```python
from build123d import *

# Parameters (mm, degrees)
SKETCH_W        = 45
SKETCH_H        = 85
PAD_DEPTH       = 10
SKETCH001_W     = 10
SKETCH001_H     = 30
PAD001_DEPTH    = 50
SKETCH002_R     = 2.5
POCKET_DEPTH    = 10
SKETCH003_R     = 2.5
POCKET001_DEPTH = 11
POCKET002_DEPTH = 5
CHAMFER_SIZE    = 17
CHAMFER001_SIZE = 2
CHAMFER002_SIZE = 5


with BuildPart() as part:
    # Sketch → Pad (new body)
    with BuildSketch(Plane.XZ):
        Rectangle(SKETCH_W, SKETCH_H)
    extrude(amount=PAD_DEPTH)

    # Sketch001 (on Face6 of Pad) → Pad001 (join)
    with BuildSketch(Plane.XZ.offset(10)):
        with Locations((-17.5, -27.5)):
            Rectangle(SKETCH001_W, SKETCH001_H)
    extrude(amount=PAD001_DEPTH)

    # Sketch002 (on Face7 of Pad001) → Pocket (cut)
    with BuildSketch(Plane(origin=(-22.5, 0, 0), x_dir=(0, 0, -1), z_dir=(-1, 0, 0))):
        with Locations((35, 52.5)):
            Circle(SKETCH002_R)
        with Locations((35, 37.5)):
            Circle(SKETCH002_R)
    extrude(amount=-POCKET_DEPTH, mode=Mode.SUBTRACT)

    # Sketch003 (on Face5 of Pocket) → Pocket001 (cut)
    with BuildSketch(Plane.XZ.offset(10)):
        with Locations((15, 35)):
            Circle(SKETCH003_R)
        with Locations((15, 20)):
            Circle(SKETCH003_R)
    extrude(amount=-POCKET001_DEPTH, mode=Mode.SUBTRACT)

    # Sketch004 (on Face4 of Pocket001) → Pocket002 (cut)
    with BuildSketch(Plane(origin=(0, 0, 0), x_dir=(1, 0, 0), z_dir=(0, 1, 0))):
        Polygon((15, -24.75), (19.113621, -22.375), (19.113621, -17.625), (15, -15.25), (10.886379, -17.625), (10.886379, -22.375), align=None)
        Polygon((19.113621, -37.375), (19.113621, -32.625), (15, -30.25), (10.886379, -32.625), (10.886379, -37.375), (15, -39.75), align=None)
    extrude(amount=-POCKET002_DEPTH, mode=Mode.SUBTRACT)

    # Chamfer
    chamfer_edges = [part.edges().sort_by_distance(p)[0] for p in [
        (22.5, -5, -42.5),
        (-22.5, -5, 42.5),
        (-17.5, -60, -12.5),
    ]]
    chamfer(chamfer_edges, length=CHAMFER_SIZE)

    # Chamfer001
    chamfer001_edges = [part.edges().sort_by_distance(p)[0] for p in [
        (-12.5, -26.5, -12.5),
        (-12.5, -51.5, -21),
        (-12.5, -60, -36),
        (-12.5, -35, -42.5),
        (22.5, 0, 8.5),
        (14, 0, -34),
        (-22.5, 0, -8.5),
        (-14, 0, 34),
        (8.5, 0, 42.5),
        (-8.5, 0, -42.5),
    ]]
    chamfer(chamfer001_edges, length=CHAMFER001_SIZE)

    # Chamfer002
    chamfer002_edges = [part.edges().sort_by_distance(p)[0] for p in [
        (-12.5, -10, -27.5),
    ]]
    chamfer(chamfer002_edges, length=CHAMFER002_SIZE)


solid = part.part
```
Verification items for the finished model (mm, model axes). A direction names the side the tool comes from. Round coordinates to 2 decimals unless told otherwise and drop trailing zeros. Order: outer loops, then holes, each group sorted by start corner. A loop starts at its lowest first (then second) coordinate and runs counter-clockwise, first axis right, second up.
1) Cross-section at B-B, the plane z = 20. Record the cut outline in (x, y), plus the area to 3 significant figures.
Geometry says:
outline: (-22.5, -10) - (12.5, -10) - (12.5, -5) - (10.89, -5) - (10.89, 0) - (-20.5, 0) - (-22.5, -2) - close; (17.5, -10) - (22.5, -10) - (22.5, -2) - (20.5, 0) - (19.11, 0) - (19.11, -5) - (17.5, -5) - close
area: 380 mm2
2) Cross-section at A-A, the plane y = -37.5. Record the cut outline in (x, z).
Geometry says:
outline: (-22.5, -42.5) - (-14.5, -42.5) - (-12.5, -40.5) - (-12.5, -37.5) - (-22.5, -37.5) - close; (-22.5, -32.5) - (-12.5, -32.5) - (-12.5, -14.5) - (-14.5, -12.5) - (-22.5, -12.5) - close
3) Cross-section at D-D, the plane z = -33.5. Record the cut outline in (x, y).
Geometry says:
outline: (-22.5, -60) - (-14.5, -60) - (-12.5, -58) - (-12.5, -54.5) - (-22.5, -54.5) - close; (-22.5, -50.5) - (-12.5, -50.5) - (-12.5, -39.5) - (-22.5, -39.5) - close; (-22.5, -35.5) - (-12.5, -35.5) - (-12.5, -15) - (-7.5, -10) - (14.5, -10) - (14.5, -2) - (11.67, 0) - (-20.5, 0) - (-22.5, -2) - close
4) Depth check by flat-ended pin: pin 1 (5 mm diameter, centred on x = 0, y = -13.5, fed in from +Z); pin 2 (10 mm diameter, centred on x = -4.5, z = 4.5, fed in from -Y); pin 3 (8 mm diameter, centred on y = -45.5, z = -29.5, fed in from +X); pin 4 (5 mm diameter, centred on y = -3.5, z = 34.5, fed in from -X). Enter the tip coordinate at first touch or a pass-through.
Geometry says:
pin 1: passes through
pin 2: stops at y = -10
pin 3: stops at x = -12.5
pin 4: stops at x = -16
5) Cross-section at C-C, the plane x = 13.5. Record the cut outline in (y, z).
Geometry says:
outline: (-10, -34.5) - (-2, -34.5) - (0, -31.67) - (0, 16.12) - (-5, 16.12) - (-5, 18) - (-10, 18) - close; (-10, 22) - (-5, 22) - (-5, 23.88) - (0, 23.88) - (0, 31.12) - (-5, 31.12) - (-5, 33) - (-10, 33) - close; (-10, 37) - (-5, 37) - (-5, 38.88) - (0, 38.88) - (0, 40.5) - (-2, 42.5) - (-10, 42.5) - close
6) Draft check along Z on faces 1 (the flat face through (14, -6, -34)), 2 (the flat face through (-13.5, -59, -36.1)), 3 (the flat face through (17.086, -2.465, 31.454)). Enter one of: +Z half, -Z half, draft (parallel to the pull), parting line (faces both ways), or undercut.
Geometry says:
face 1: -Z half
face 2: draft
face 3: undercut
7) Tool access check on faces 4 (the flat face through (-14, -6, 34)), 5 (the flat face through (-13, -23, -14)), 6 (the flat face through (10.886, -2, 35)). Record the directions out of +Z, -Z, +X, -X, +Y, -Y that give a thin tool (end or side, any length) a straight path to the whole face; none if there is none.
Geometry says:
face 4: +Z, -X, +Y, -Y
face 5: +Z, +X, -Y
face 6: +Y
8) Material ranges on line 1 (Y direction, x = -15.5, z = -35); line 2 (Y direction, x = -11, z = -3.5); line 3 (Z direction, x = -18, y = -27.5), recorded low to high.
Geometry says:
line 1: y = -60 to -55, -50 to -40, -35 to 0
line 2: y = -10 to 0
line 3: z = -42.5 to -12.5
